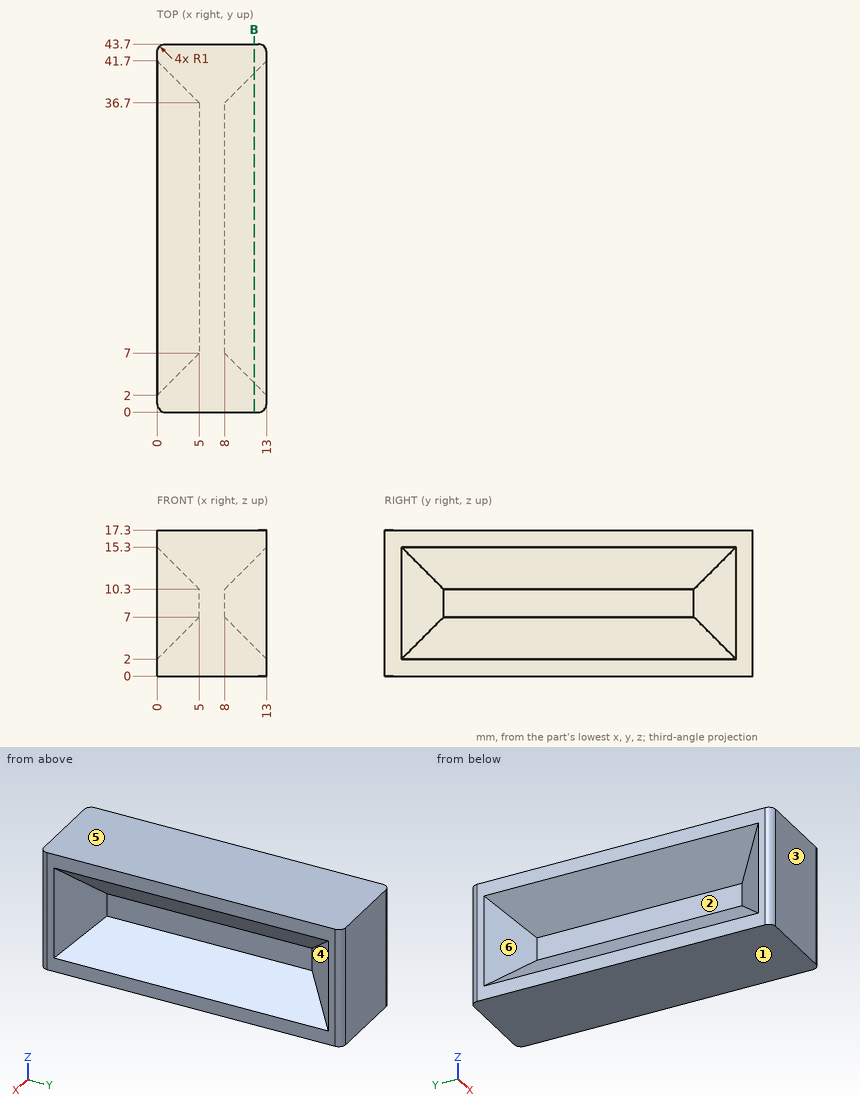
Verification items for this drawing (mm, ordinates from the low corner). A direction names the side the tool comes from. Coordinates: 2 decimals unless noted, no trailing zeros. Write each loop counter-clockwise with the first axis right and the second up, starting at its lowest first coordinate (ties: lowest second). Pieces come first, ordered by that corner, then holes. Notation, with made-up numbers: M 83.25,63 L 122.25,63 A34 ccw 122.25,101 Z; hole C 85,48 d4. An arc over 180 degrees is marked long. Answer as a JSON object with one key per item and string values.
1. Tool access check on the marked faces 4, 5 and 6. Record the directions out of +Z, -Z, +X, -X, +Y, -Y that give a thin tool (end or side, any length) a straight path to the whole face; none if there is none.
Answers below:
{"face 4": "+X", "face 5": "+Z, +X, -X, +Y, -Y", "face 6": "-X"}
2. Scan lines: L1, parallel to Z at x = 8.25, y = 24; L2, parallel to Z at x = 9, y = 24.5; L3, parallel to Y at x = 12.25, z = 10.25. Record each from-to range of solid material in increasing order.
Answers below:
{"L1": "z = 0 to 6.75, 10.55 to 17.3", "L2": "z = 0 to 6, 11.3 to 17.3", "L3": "y = 0.03 to 2.75, 40.95 to 43.67"}
3. Section check B-B, the plane x = 11.5. Enter the section's corners in (y, z), plus the area to 3 significant figures.
Answers below:
{"outline": "M 0,0 L 43.7,0 L 43.7,17.3 L 0,17.3 Z; hole M 3.5,3.5 L 40.2,3.5 L 40.2,13.8 L 3.5,13.8 Z", "area": "378 mm²"}
4. Go/stop test with flat-tipped pins: pin 1 Ø1 at (y, z) = (21, 8) entering from -X; pin 2 Ø1.5 at (y, z) = (22.5, 11) entering from +X; pin 3 Ø8 at (y, z) = (24, 11) entering from +X. Record where each tip stops, or that it passes through.
Answers below:
{"pin 1": "stops at x = 5", "pin 2": "stops at x = 9.45", "pin 3": "stops at x = 12.7"}
5. Draft check along Y on the marked faces 1, 2 and 3. Enter one of: released by +Y, released by -Y, zero draft, split by the parting line, or undercut.
Answers below:
{"face 1": "zero draft", "face 2": "undercut", "face 3": "released by -Y"}
